```python
from build123d import *

# Parameters (mm, degrees)
BOSS_EXTRUDE1_DEPTH = 10
SKETCH2_R           = 1.7
CUT_EXTRUDE1_DEPTH  = 20.805330599


with BuildPart() as part:
    # Sketch1 → Boss-Extrude1 (new body)
    with BuildSketch(Plane.XY):
        with BuildLine():
            Line((4.06124537, -3.927452752), (4.06124537, -5.854221643))
            ThreePointArc((4.06124537, -5.854221643), (6.312764777, -3.303729085), (7.125, 0))
            ThreePointArc((7.125, 0), (-3.303729085, 6.312764777), (-4.06124537, -5.854221643))
            Line((-4.06124537, -5.854221643), (-4.06124537, -3.927452752))
            Line((-4.06124537, -3.927452752), (-1.26124537, -3.927452752))
            ThreePointArc((-1.26124537, -3.927452752), (-2.430327946, 3.333036315), (4.125, 0))
            ThreePointArc((4.125, 0), (3.333036315, -2.430327946), (1.26124537, -3.927452752))
            Line((1.26124537, -3.927452752), (4.06124537, -3.927452752))
        make_face()
        with BuildLine():
            ThreePointArc((-4.06124537, -5.854221643), (-2.723530413, -6.583920343), (-1.26124537, -7.012480668))
            Line((-1.26124537, -7.012480668), (-1.26124537, -3.927452752))
            Line((-1.26124537, -3.927452752), (-4.06124537, -3.927452752))
            Line((-4.06124537, -3.927452752), (-4.06124537, -5.854221643))
        make_face()
        with BuildLine():
            Line((1.26124537, -3.927452752), (1.26124537, -7.012480668))
            ThreePointArc((1.26124537, -7.012480668), (2.723530413, -6.583920343), (4.06124537, -5.854221643))
            Line((4.06124537, -5.854221643), (4.06124537, -3.927452752))
            Line((4.06124537, -3.927452752), (1.26124537, -3.927452752))
        make_face()
        with BuildLine():
            Line((1.26124537, -7.012480668), (1.26124537, -12.927452752))
            Line((1.26124537, -12.927452752), (4.06124537, -12.927452752))
            Line((4.06124537, -12.927452752), (4.06124537, -5.854221643))
            ThreePointArc((4.06124537, -5.854221643), (2.723530413, -6.583920343), (1.26124537, -7.012480668))
        make_face()
        with BuildLine():
            Line((-1.26124537, -12.927452752), (-1.26124537, -7.012480668))
            ThreePointArc((-1.26124537, -7.012480668), (-2.723530413, -6.583920343), (-4.06124537, -5.854221643))
            Line((-4.06124537, -5.854221643), (-4.06124537, -12.927452752))
            Line((-4.06124537, -12.927452752), (-1.26124537, -12.927452752))
        make_face()
    extrude(amount=BOSS_EXTRUDE1_DEPTH)

    # Sketch2 → Cut-Extrude1 (cut, through all)
    with BuildSketch(Plane.ZY.offset(4.06124537)):
        with Locations(Location((5, -9.390837197, 0), (0, 0, 270))):
            Circle(SKETCH2_R)
    extrude(amount=-CUT_EXTRUDE1_DEPTH, mode=Mode.SUBTRACT)


solid = part.part
```
Geometry: final body of the model. Coordinates: model frame, mm. A direction names the side the tool comes from. Round coordinates to 2 decimals unless told otherwise and drop trailing zeros. Order: outer loops, then holes, each group sorted by start corner. A loop starts at its lowest first (then second) coordinate and runs counter-clockwise, first axis right, second up. Notation, with made-up numbers: (-22.5, 66.5) -> (-6.5, 66.5) arc R21 cw to (-6.5, 94.5) -> close; hole circle Ø6 at (54.5, -19.75). An arc over 180 degrees is marked (long way). Use one line per item in the form item = value. Start each with the question number.
1. Cut plane A-A (x = -2). Return the cut outline in (y, z), then the cut area to 3 significant figures.
2. Line query: probe 1 along X at (y, z) = (-6.75, 5.75); probe 2 along Y at (x, z) = (1.5, 8.75); probe 3 along Y at (x, z) = (-3.75, 6.25). Output: solid intervals per line, ascending.
3. Cut plane D-D (x = 0). Return the cut outline in (y, z) (3 decimals).
4. Cut plane B-B (z = 5). Return the cut outline in (x, y) (3 decimals), then the cut area to 3 significant figures.
5. Pin query (flat end, axial travel): pin 1 Ø2 at (x, z) = (3.5, 3) entering from +Y; pin 2 Ø3 at (y, z) = (-5, 8) entering from -X; pin 3 Ø4 at (y, z) = (4, 3) entering from +X; pin 4 Ø2 at (y, z) = (-9.39, 5) entering from +X. Return the tip coordinate at first contact, or that it passes through.
6. Cut plane C-C (z = 7.5). Return the cut outline in (x, y) (3 decimals).
7. Draft query along X for faces 4 (the face through (1.5, -5, 0)), 5 (the face through (-4.061, -7.8, 3.8)), 6 (the face through (1.261, -7, 5)). Return one class per face: pulls with the +X half, pulls with the -X half, needs draft (parallel to the pull), parting line crosses it, or undercut.
8. Reachability of faces 1 (the face through (-1.261, -7, 5)), 2 (the face through (4.061, -7.9, 3.8)), 3 (the face through (2.64, -8.04, 3.97)) from +Z, -Z, +X, -X, +Y, -Y: full face, straight path, thin tool, end or side. Return the list, or none.
Solution:
q1.outline = (-12.93, 0) -> (-3.61, 0) -> (-3.61, 10) -> (-12.93, 10) -> close; (3.61, 0) -> (6.84, 0) -> (6.84, 10) -> (3.61, 10) -> close; hole circle Ø3.4 at (-9.39, 5)
q1.area = 116 mm^2
q2.probe_1 = -4.06 to -1.26, 1.26 to 4.06
q2.probe_2 = -12.93 to -3.84, 3.84 to 6.97
q2.probe_3 = -12.93 to -10.54, -8.24 to -1.72, 1.72 to 6.06
q3.outline = (4.125, 0) -> (7.125, 0) -> (7.125, 10) -> (4.125, 10) -> close
q4.outline = (-4.061, -12.927) -> (-1.261, -12.927) -> (-1.261, -11.091) -> (-4.061, -11.091) -> close; (-4.061, -7.691) -> (-1.261, -7.691) -> (-1.261, -3.927) arc R4.125 cw (long way) to (1.261, -3.927) -> (1.261, -7.691) -> (4.061, -7.691) -> (4.061, -5.854) arc R7.125 ccw (long way) to (-4.061, -5.854) -> close; (1.261, -12.927) -> (4.061, -12.927) -> (4.061, -11.091) -> (1.261, -11.091) -> close
q4.area = 115 mm^2
q5.pin_1 = 6.67
q5.pin_2 = -6.21
q5.pin_3 = 6.84
q5.pin_4 = through
q6.outline = (-4.061, -12.927) -> (-1.261, -12.927) -> (-1.261, -3.927) arc R4.125 cw (long way) to (1.261, -3.927) -> (1.261, -12.927) -> (4.061, -12.927) -> (4.061, -5.854) arc R7.125 ccw (long way) to (-4.061, -5.854) -> close
q7.face_4 = needs draft
q7.face_5 = pulls with the -X half
q7.face_6 = undercut
q8.face_1 = +Z, -Z, -Y
q8.face_2 = +Z, -Z, +X, -Y
q8.face_3 = +X, -X
